Autodesk Inventor part; units mm, degrees
ref_plane "YZ Plane" through (0, 0, 0) normal (1, 0, 0) x (0, 1, 0)
ref_plane "XZ Plane" through (0, 0, 0) normal (0, 1, 0) x (-1, 0, 0)
ref_plane "XY Plane" through (0, 0, 0) normal (0, 0, 1) x (1, 0, 0)
sketch "Sketch1" plane through (0, 0, 0) normal (0, 1, 0) x (-1, 0, 0)
  line L0 (93.6212, 93.2037) -> (93.6212, -131.4276) construction
  line L1 (93.6212, -131.4276) -> (12.1295, -131.4276) construction
  line L2 (12.1295, -131.4276) -> (12.1295, 93.2037) construction
  line L3 (12.1295, 93.2037) -> (93.6212, 93.2037) construction
  circle A0 centre (0, 0) radius 13.9
  circle A1 centre (0, 0) radius 8 construction
  circle A2 centre (0, 0) radius 9.5 construction
  line L4 (0, 0) -> (-9.8288, -9.8288) construction
  line L5 (0, 0) -> (13.9, 0) construction
  line L6 (0, 0) -> (9.8288, -9.8288) construction
  line L7 (0, 0) -> (9.8288, 9.8288) construction
  line L8 (0, 0) -> (-9.8288, 9.8288) construction
  point P0 (-6.7175, 6.7175)
  point P1 (-5.6569, -5.6569)
  point P2 (6.7175, -6.7175)
  point P3 (5.6569, 5.6569)
  dimension "d7" = 27.8
  dimension "d8" = 16
  dimension "d9" = 19
  dimension "d10" = 135
extrude "Extrusion1" add sketch "Sketch1" along normal blind 24
hole "Hole1" at (6.7175, 0, 6.7175) at (5.6569, 0, -5.6569) at (-6.7175, 0, -6.7175) at (-5.6569, 0, 5.6569) direction (0, 1, 0) diameter 3 depth 4
sketch "Sketch2" plane through (0, 24, 0) normal (0, 1, 0) x (1, 0, 0)
  circle A0 centre (0, 0) radius 3
  dimension "d25" = 6
extrude "Extrusion2" add sketch "Sketch2" along normal blind 14
properties part number "MOTOR"
For this review, take the finished solid that the model builds, in its own axes (mm). A direction names the side the tool comes from. Coordinates: 2 decimals unless noted, no trailing zeros. Write each loop counter-clockwise with the first axis right and the second up, starting at its lowest first coordinate (ties: lowest second). Pieces come first, ordered by that corner, then holes.
(1) For pin 1 Ø4 at (x, y) = (-6.5, 15.5) entering from +Z; pin 2 Ø1.5 at (x, z) = (-5, 5.5) entering from -Y; pin 3 Ø5 at (x, z) = (-4, 8.5) entering from +Y, all flat-tipped, find the tip position at first contact; note any pin that passes through.
(2) Add section B-B on x = 0. Give the boundary of the cut face in (y, z), then the cut area to 3 significant figures.
(3) Add section C-C on y = 25. Give the boundary of the cut face in (x, z).
(4) Wall thickness on probe 1 along Y at (x, z) = (-11.75, -4.25); probe 2 along Z at (x, y) = (0, 16.5); probe 3 along X at (y, z) = (33, -2.5): over which ranges is each line inside the solid? List them lowest first.
(5) Tool access review of faces 5 (the face through (-7, 4, -7)), 6 (the face through (3.01, 11.83, 13.57)): name each direction out of +Z, -Z, +X, -X, +Y, -Y from which nothing blocks a thin tool from reaching the whole face with its end or side.
(6) The part is to be moulded in two halves that separate along X. For faces 1 (the face through (0.2, 24, 3.3)), 2 (the face through (-6, 4, 6)), 3 (the face through (-3, 31, 0)), 4 (the face through (6, 4, -6)), say which applies: +X half, -X half, draft (parallel to the pull), parting line (faces both ways), or undercut.
(7) Add section D-D on z = 5.75. Give the boundary of the cut face in (x, y).
(8) Add section A-A on z = 0. Give the boundary of the cut face in (x, y).
Answer sheet:
1. pin 1: stops at z = 13.15
1. pin 2: stops at y = 4
1. pin 3: stops at y = 24
2. outline: (0, -13.9) - (24, -13.9) - (24, -3) - (38, -3) - (38, 3) - (24, 3) - (24, 13.9) - (0, 13.9) - close
2. area: 751 mm2
3. outline: circle Ø6 at (0, 0)
4. probe 1: y = 0 to 24
4. probe 2: z = -13.9 to 13.9
4. probe 3: x = -1.66 to 1.66
5. face 5: -Y
5. face 6: +Y, -Y
6. face 1: draft
6. face 2: undercut
6. face 3: parting line
6. face 4: undercut
7. outline: (-12.65, 0) - (-7.15, 0) - (-7.15, 4) - (-4.16, 4) - (-4.16, 0) - (5.57, 0) - (5.57, 4) - (7.86, 4) - (7.86, 0) - (12.65, 0) - (12.65, 24) - (-12.65, 24) - close
8. outline: (-13.9, 0) - (13.9, 0) - (13.9, 24) - (3, 24) - (3, 38) - (-3, 38) - (-3, 24) - (-13.9, 24) - close
